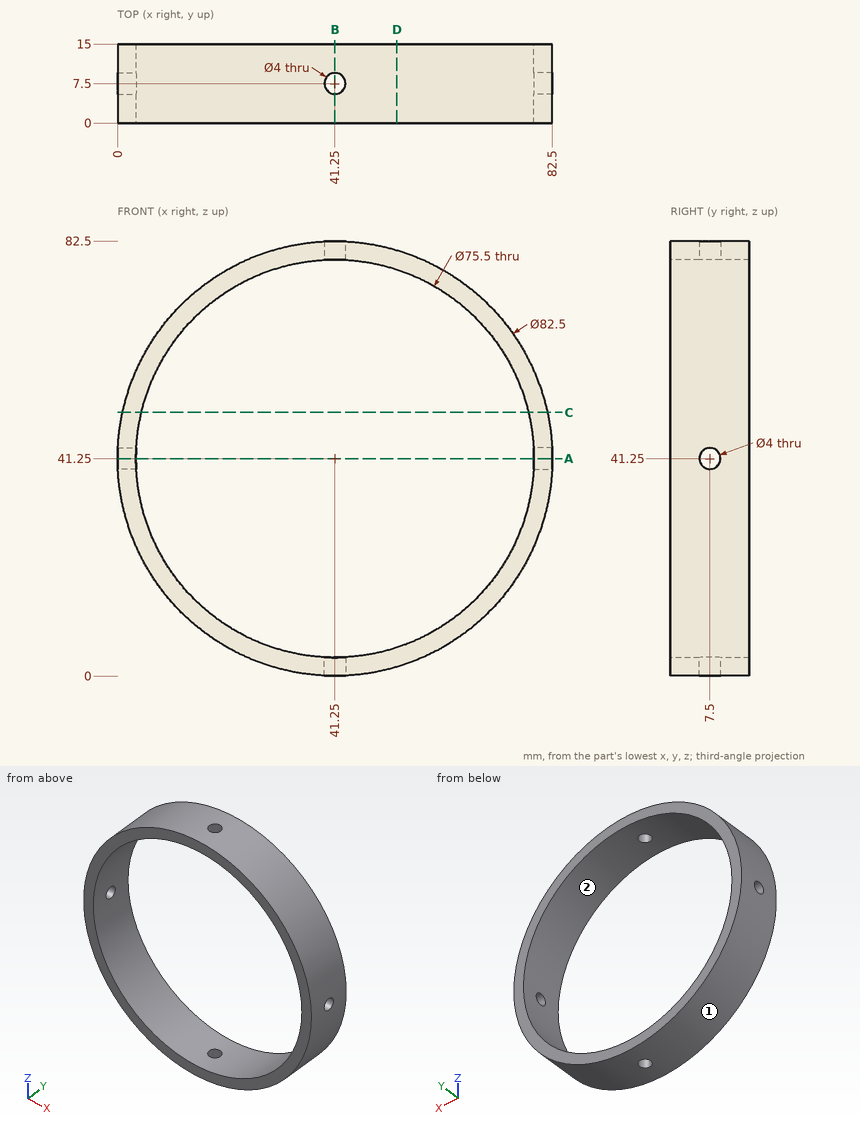
Geometry: see drawing. Coordinates: mm, zero at the bounding-box minimum. Round coordinates to 2 decimals unless told otherwise and drop trailing zeros. Write each loop counter-clockwise with the first axis right and the second up, starting at its lowest first coordinate (ties: lowest second). Pieces come first, ordered by that corner, then holes.
Item 1: Material intervals for L1, parallel to Y at x = 2, z = 41; L2, parallel to X at y = 10, z = 55; L3, parallel to Z at x = 59, y = 3, sorted ascending.
Item 2: Section query B-B (x = 41.25). Return loops of the section in (y, z).
Item 3: Pin query (flat end, axial travel): P1, Ø2, axis at x = 40, y = 2, coming from the +Z side; P2, Ø4, axis at y = 10, z = 60, coming from the +X side; P3, Ø6, axis at x = 53, y = 13.5, coming from the -Z side. Return the tip coordinate at first contact, or that it passes through.
Item 4: Section query D-D (x = 53). Return loops of the section in (y, z).
Item 5: Section query A-A (z = 41.25). Return loops of the section in (x, y), plus the area to 3 significant figures.
Item 6: Mould query, pull axis X, two halves, no side actions, for the marked faces 1 and 2. Classes: +X half, -X half, draft (parallel to the pull), parting line (faces both ways), or undercut.
Item 7: Section query C-C (z = 50). Return loops of the section in (x, y).
Completed:
1. L1: y = 0 to 5.52, 9.48 to 15
1. L2: x = 2.36 to 6.09, 76.41 to 80.14
1. L3: z = 4.01 to 7.93, 74.57 to 78.49
2. outline: (0, 0) - (5.5, 0) - (5.5, 3.5) - (0, 3.5) - close; (0, 79) - (5.5, 79) - (5.5, 82.5) - (0, 82.5) - close; (9.5, 0) - (15, 0) - (15, 3.5) - (9.5, 3.5) - close; (9.5, 79) - (15, 79) - (15, 82.5) - (9.5, 82.5) - close
3. P1: stops at z = 82.5
3. P2: stops at x = 78.95
3. P3: stops at z = 0.94
4. outline: (0, 1.71) - (15, 1.71) - (15, 5.38) - (0, 5.38) - close; (0, 77.12) - (15, 77.12) - (15, 80.79) - (0, 80.79) - close
5. outline: (0, 0) - (3.5, 0) - (3.5, 5.5) - (0, 5.5) - close; (0, 9.5) - (3.5, 9.5) - (3.5, 15) - (0, 15) - close; (79, 0) - (82.5, 0) - (82.5, 5.5) - (79, 5.5) - close; (79, 9.5) - (82.5, 9.5) - (82.5, 15) - (79, 15) - close
5. area: 77.0 mm2
6. face 1: parting line
6. face 2: undercut
7. outline: (0.94, 0) - (4.53, 0) - (4.53, 15) - (0.94, 15) - close; (77.97, 0) - (81.56, 0) - (81.56, 15) - (77.97, 15) - close
